Can you work these out from the model? Positions are in its coordinate system, mm. Face numbers are marked on the shaded views. A direction names the side the tool comes from. Round coordinates to 2 decimals unless told otherwise and drop trailing zeros. Loops run counter-clockwise (first coordinate to the right, second up) from the corner with the lowest first, then second, coordinate; pieces in that order, holes last. Notation, with made-up numbers: M 80,1.25 L 94,1.25 A19 cw 94,37.25 Z; hole C -25,27 d5. An arc over 180 degrees is marked long. Return JSON: item names as keys, results as strings.
```python
from build123d import *

# Parameters (mm, degrees)
SKETCH2_W           = 23.8
SKETCH2_H           = 18.9
BOSS_EXTRUDE1_DEPTH = 31.6
SHELL2_T            = -2
SKETCH10_W          = 21.8
SKETCH10_H          = 1
CUT_EXTRUDE5_DEPTH  = 24.8
SKETCH12_R          = 2.95
CUT_EXTRUDE6_DEPTH  = 2


with BuildPart() as part:
    # Sketch2 → Boss-Extrude1 (new body)
    with BuildSketch(Plane(origin=(-2.162079654, 0, 0), x_dir=(1, 0, 0), z_dir=(0, 1, 0))):
        with Locations((-82.717170842, -18.240014695)):
            Rectangle(SKETCH2_W, SKETCH2_H)
    extrude(amount=BOSS_EXTRUDE1_DEPTH)

    # Shell2
    shell2_openings = [part.faces().sort_by_distance(p)[0] for p in [
        (-84.879250496, 15.8, 27.690014695),
    ]]
    offset(amount=SHELL2_T, openings=shell2_openings, kind=Kind.INTERSECTION)

    # Sketch10 → Cut-Extrude5 (cut)
    with BuildSketch(Plane.XZ):
        with Locations((-84.938526567, 26.190014695)):
            Rectangle(SKETCH10_W, SKETCH10_H)
    extrude(amount=-CUT_EXTRUDE5_DEPTH, mode=Mode.SUBTRACT)

    # Sketch12 → Cut-Extrude6 (cut)
    with BuildSketch(Plane(origin=(0, 0, 0), x_dir=(-1, 0, 0), z_dir=(0, -1, 0))):
        with Locations(Location((84.879250496, -18.240014695, 0), (0, 0, 90))):
            Circle(SKETCH12_R)
    extrude(amount=-CUT_EXTRUDE6_DEPTH, mode=Mode.SUBTRACT)


solid = part.part
```
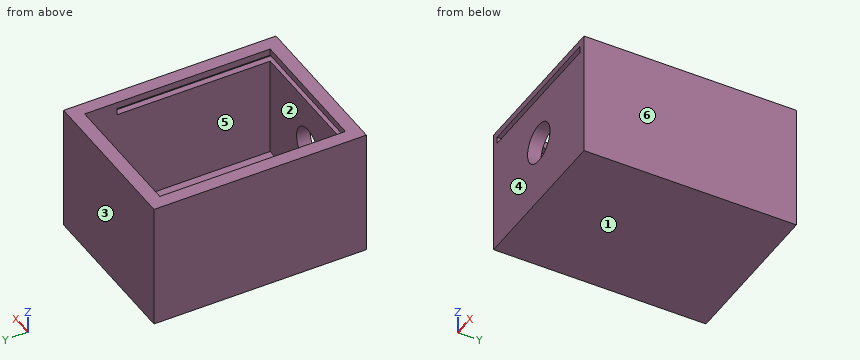
Q1. Suppose I cut it at D-D, the plane x = -83.75. Please give me the cut outline in (y, z).
Results:
{"outline": "M 0,8.79 L 31.6,8.79 L 31.6,27.69 L 29.6,27.69 L 29.6,10.79 L 2,10.79 L 2,15.51 L 0,15.51 Z; M 0,20.97 L 2,20.97 L 2,25.69 L 0,25.69 Z; M 0,26.69 L 2,26.69 L 2,27.69 L 0,27.69 Z"}
Q2. Suppose I cut it at C-C, the plane y = 18. Please give me the cut outline in (x, z).
Results:
{"outline": "M -96.78,8.79 L -72.98,8.79 L -72.98,27.69 L -74.98,27.69 L -74.98,26.69 L -74.04,26.69 L -74.04,25.69 L -74.98,25.69 L -74.98,10.79 L -94.78,10.79 L -94.78,25.69 L -95.84,25.69 L -95.84,26.69 L -94.78,26.69 L -94.78,27.69 L -96.78,27.69 Z"}
Q3. On a 3-axis mill with a long thin cutter (end or side, diameter ignored), from which of +Z, -Z, +X, -X, +Y, -Y can I reach the whole of each face in a straight line? I mean the marked faces 5 and 6. Say none if no direction works.
Results:
{"face 5": "+Z", "face 6": "+Z, -Z, +X, +Y, -Y"}
Q4. I'm going to push a flat-ended pin straight in: pin 1 Ø6.5 at (x, y) = (-89.5, 8.5) entering from +Z. Where does the tip first touch, or does it pass through?
Results:
{"pin 1": "stops at z = 10.79"}
Q5. Suppose I cut it at A-A, the plane z = 14.25. Please give me the cut outline in (x, y).
Results:
{"outline": "M -96.78,0 L -72.98,0 L -72.98,31.6 L -96.78,31.6 Z; hole M -94.78,2 L -74.98,2 L -74.98,29.6 L -94.78,29.6 Z"}
Q6. Suppose I cut it at B-B, the plane x = -92.75. Please give me the cut outline in (y, z), plus the area to 3 significant figures.
Results:
{"outline": "M 0,8.79 L 31.6,8.79 L 31.6,27.69 L 29.6,27.69 L 29.6,10.79 L 2,10.79 L 2,25.69 L 0,25.69 Z; M 0,26.69 L 2,26.69 L 2,27.69 L 0,27.69 Z", "area": "129 mm2"}
Q7. Thinking about a two-plate mould opening in Y: for the marked faces 1, 2, 3 and 4, which applies, pulls with the +Y half, pulls with the -Y half, needs draft (parallel to the pull), parting line crosses it, or undercut?
Results:
{"face 1": "needs draft", "face 2": "undercut", "face 3": "pulls with the +Y half", "face 4": "pulls with the -Y half"}
Q8. If I drill on line 1 along X through (y, z) = (7.5, 16); line 2 along Y through (x, z) = (-93.75, 14); line 3 along Z through (x, y) = (-84, 5), over which ranges is the centre line in solid material (lowest first)?
Results:
{"line 1": "x = -96.78 to -94.78, -74.98 to -72.98", "line 2": "y = 0 to 2, 29.6 to 31.6", "line 3": "z = 8.79 to 10.79"}
